from build123d import *

# Parameters (mm, degrees)
SKETCH1_R                = 57.5
SKETCH1_R_2              = 1.89865
SKETCH1_R_3              = 1.9939
SKETCH1_R_4              = 8
BOSS_EXTRUDE1_DEPTH      = 6.35
CUT_EXTRUDE1_DEPTH       = 82.564836173
SKETCH3_W                = 6.35
SKETCH3_H                = 80
CUT_EXTRUDE3_DEPTH       = 82.564836173
CUT_EXTRUDE4_DEPTH       = 82.564836173
CUT_EXTRUDE6_DEPTH       = 82.564836173
FILLET1_R                = 2
CIRPATTERN1_COUNT        = 8
FILLET1_OF_CIRPATTERN1_R = 2
CUT_EXTRUDE7_DEPTH       = 10
FILLET2_R                = 2
CIRPATTERN2_COUNT        = 8
FILLET2_OF_CIRPATTERN2_R = 2


with BuildPart() as part:
    # Sketch1 → Boss-Extrude1 (new body)
    with BuildSketch(Plane.XY):
        Circle(SKETCH1_R)
        with Locations((45.315389352, 21.130913087)):
            Circle(SKETCH1_R_2, mode=Mode.SUBTRACT)
        with Locations((46.467376211, -18.460307366)):
            Circle(SKETCH1_R_3, mode=Mode.SUBTRACT)
        Circle(SKETCH1_R_4, mode=Mode.SUBTRACT)
        with Locations((49.978847504, 1.454235937)):
            Circle(SKETCH1_R_3, mode=Mode.SUBTRACT)
        with Locations((0, -40)):
            Circle(SKETCH1_R_3, mode=Mode.SUBTRACT)
        with Locations((0, -50)):
            Circle(SKETCH1_R_2, mode=Mode.SUBTRACT)
        with Locations((-28.284271247, -28.284271247)):
            Circle(SKETCH1_R_3, mode=Mode.SUBTRACT)
        with Locations((-35.355339059, -35.355339059)):
            Circle(SKETCH1_R_2, mode=Mode.SUBTRACT)
        with Locations((-40, 0)):
            Circle(SKETCH1_R_3, mode=Mode.SUBTRACT)
        with Locations((-50, 0)):
            Circle(SKETCH1_R_2, mode=Mode.SUBTRACT)
        with Locations((-28.284271247, 28.284271247)):
            Circle(SKETCH1_R_3, mode=Mode.SUBTRACT)
        with Locations((-35.355339059, 35.355339059)):
            Circle(SKETCH1_R_2, mode=Mode.SUBTRACT)
        with Locations((0, 40)):
            Circle(SKETCH1_R_3, mode=Mode.SUBTRACT)
        with Locations((0, 50)):
            Circle(SKETCH1_R_2, mode=Mode.SUBTRACT)
        with Locations((35.355339059, -35.355339059)):
            Circle(SKETCH1_R_2, mode=Mode.SUBTRACT)
    extrude(amount=BOSS_EXTRUDE1_DEPTH)

    # Sketch2 → Cut-Extrude1 (cut, through all)
    with BuildSketch(Plane.XY):
        Polygon((12.5, -29.35), (41, -29.35), (41, 10.65), (44.5, 10.65), (44.5, 17), (41, 17), (41, 32), (21, 32), (21, 17), (17.5, 17), (17.5, 10.65), (21, 10.65), (21, 5.65), (12.5, 5.65), align=None)
    extrude(amount=CUT_EXTRUDE1_DEPTH, mode=Mode.SUBTRACT)

    # Sketch3 → Cut-Extrude3 (cut, through all)
    with BuildSketch(Plane.XY.offset(6.35)):
        with Locations((31, 32)):
            Rectangle(SKETCH3_W, SKETCH3_H)
    extrude(amount=-CUT_EXTRUDE3_DEPTH, mode=Mode.SUBTRACT)

    # Sketch4 → Cut-Extrude4 (cut, through all)
    with BuildSketch(Plane.XY.offset(6.35)):
        with BuildLine():
            Line((21, -36.5), (21, -16.443021443))
            Line((21, -16.443021443), (24.175, -16.470277755))
            Line((24.175, -16.470277755), (24.175, -57.5))
            Line((24.175, -57.5), (0, -57.5))
            ThreePointArc((0, -57.5), (14.849242405, -51.349242405), (21, -36.5))
        make_face()
        with BuildLine():
            Line((0, 57.5), (24.175, 57.5))
            Line((24.175, 57.5), (24.175, 16.470277755))
            Line((24.175, 16.470277755), (21, 16.443021443))
            Line((21, 16.443021443), (21, 36.5))
            ThreePointArc((21, 36.5), (14.849242405, 51.349242405), (0, 57.5))
        make_face()
    extrude(amount=-CUT_EXTRUDE4_DEPTH, mode=Mode.SUBTRACT)


with BuildPart() as cut_extrude4_kept_piece:
    # of the separate pieces the step leaves, the one the design keeps (cut_extrude4_pieces_kept)
    add(part.part.solids().sort_by_distance((0, 57.5, 0))[0])

    # Sketch6 → Cut-Extrude6 (cut, through all)
    with BuildSketch(Plane.XY.offset(6.35)):
        with BuildLine():
            Line((-13.691998588, 3.668759964), (-32.503404055, 8.709260868))
            ThreePointArc((-32.503404055, 8.709260868), (-33.65, 0), (-32.503404055, -8.709260868))
            Line((-32.503404055, -8.709260868), (-13.691998588, -3.668759964))
            ThreePointArc((-13.691998588, -3.668759964), (-14.175, 0), (-13.691998588, 3.668759964))
        make_face()
    cut_extrude6 = extrude(amount=-CUT_EXTRUDE6_DEPTH, mode=Mode.SUBTRACT)

    # Fillet1
    fillet1_edges = [cut_extrude4_kept_piece.edges().sort_by_distance(p)[0] for p in [
        (-13.691998588, 3.668759964, 3.175),
        (-13.691998588, -3.668759964, 3.175),
        (-32.503404055, -8.709260868, 3.175),
        (-32.503404055, 8.709260868, 3.175),
    ]]
    fillet(fillet1_edges, radius=FILLET1_R)

    # CirPattern1: Cut-Extrude6 ×8 about axis, 3 skipped
    cirpattern1_axis = Axis((0, 0, 0), (0, 0, -1))
    add([cut_extrude6.rotate(cirpattern1_axis, i * 360 / CIRPATTERN1_COUNT) for i in range(1, CIRPATTERN1_COUNT) if i not in (3, 4, 5)], mode=Mode.SUBTRACT)

    # Fillet1 of CirPattern1
    fillet1_of_cirpattern1_edges = [cut_extrude4_kept_piece.edges().sort_by_distance(p)[0] for p in [
        (-7.0875, 12.275910099, 3.175),
        (-12.275910099, 7.0875, 3.175),
        (-29.141754837, 16.825, 3.175),
        (-16.825, 29.141754837, 3.175),
        (3.668759964, 13.691998588, 3.175),
        (-3.668759964, 13.691998588, 3.175),
        (-8.709260868, 32.503404055, 3.175),
        (8.709260868, 32.503404055, 3.175),
        (-3.668759964, -13.691998588, 3.175),
        (3.668759964, -13.691998588, 3.175),
        (8.709260868, -32.503404055, 3.175),
        (-8.709260868, -32.503404055, 3.175),
        (-12.275910099, -7.0875, 3.175),
        (-7.0875, -12.275910099, 3.175),
        (-16.825, -29.141754837, 3.175),
        (-29.141754837, -16.825, 3.175),
    ]]
    fillet(fillet1_of_cirpattern1_edges, radius=FILLET1_OF_CIRPATTERN1_R)

    # Sketch7 → Cut-Extrude7 (cut)
    with BuildSketch(Plane.XY.offset(6.35)):
        with BuildLine():
            Line((-43.098920211, 33.070964631), (-29.215236756, 22.417639623))
            ThreePointArc((-29.215236756, 22.417639623), (-34.021863785, 14.092317397), (-36.50995702, 4.806627029))
            Line((-36.50995702, 4.806627029), (-53.860242094, 7.090835392))
            ThreePointArc((-53.860242094, 7.090835392), (-50.189755604, 20.789277463), (-43.098920211, 33.070964631))
        make_face()
    cut_extrude7 = extrude(amount=-CUT_EXTRUDE7_DEPTH, mode=Mode.SUBTRACT)

    # Fillet2
    fillet2_edges = [cut_extrude4_kept_piece.edges().sort_by_distance(p)[0] for p in [
        (-29.215236756, 22.417639623, 3.175),
        (-36.50995702, 4.806627029, 3.175),
        (-53.860242094, 7.090835392, 3.175),
        (-43.098920211, 33.070964631, 3.175),
    ]]
    fillet(fillet2_edges, radius=FILLET2_R)

    # CirPattern2: Cut-Extrude7 ×8 about axis, 4 skipped
    cirpattern2_axis = Axis((0, 0, 0), (0, 0, -1))
    add([cut_extrude7.rotate(cirpattern2_axis, i * 360 / CIRPATTERN2_COUNT) for i in range(1, CIRPATTERN2_COUNT) if i not in (2, 3, 4, 5)], mode=Mode.SUBTRACT)

    # Fillet2 of CirPattern2
    fillet2_of_cirpattern2_edges = [cut_extrude4_kept_piece.edges().sort_by_distance(p)[0] for p in [
        (-4.806627029, 36.50995702, 3.175),
        (-22.417639623, 29.215236756, 3.175),
        (-33.070964631, 43.098920211, 3.175),
        (-7.090835392, 53.860242094, 3.175),
        (-22.417639623, -29.215236756, 3.175),
        (-4.806627029, -36.50995702, 3.175),
        (-7.090835392, -53.860242094, 3.175),
        (-33.070964631, -43.098920211, 3.175),
        (-36.50995702, -4.806627029, 3.175),
        (-29.215236756, -22.417639623, 3.175),
        (-43.098920211, -33.070964631, 3.175),
        (-53.860242094, -7.090835392, 3.175),
    ]]
    fillet(fillet2_of_cirpattern2_edges, radius=FILLET2_OF_CIRPATTERN2_R)


solid = cut_extrude4_kept_piece.part
Input: part model. Units: mm. Frame: model coordinates. A direction names the side the tool comes from. Round coordinates to 2 decimals unless told otherwise and drop trailing zeros. Order: outer loops, then holes, each group sorted by start corner. A loop starts at its lowest first (then second) coordinate and runs counter-clockwise, first axis right, second up. Notation, with made-up numbers: (84.5, -25.5) - (92.5, -25.5) arc R21 cw to (92.5, -16.5) - close; hole circle Ø5 at (38, 48.5). An arc over 180 degrees is marked (long way). Use a Markdown table: item, result.
1. First-contact query: pin 1 (1.9 mm diameter, centred on y = 14.5, z = 2.5, fed in from +X); pin 2 (1.9 mm diameter, centred on x = 17.5, z = 2, fed in from -Y); pin 3 (1.5 mm diameter, centred on x = -9.5, z = 3, fed in from -Y). Flat tips, straight axial feed; report the tip coordinate or a pass-through.
Evaluation:
| item | result |
|---|---|
| pin 1 | x = 17.5 |
| pin 2 | y = -49.43 |
| pin 3 | y = -56.83 |
2. Section A-A on y = -40. Return the cut outline in (x, z).
Evaluation:
| item | result |
|---|---|
| outline | (-41.31, 0) - (-30.69, 0) - (-30.69, 6.35) - (-41.31, 6.35) - close; (-5.27, 0) - (-1.99, 0) - (-1.99, 6.35) - (-5.27, 6.35) - close; (1.99, 0) - (20.71, 0) - (20.71, 6.35) - (1.99, 6.35) - close |
3. Access query for faces 1 (the face through (17.5, 14, 3)), 2 (the face through (-5.955, 45.234, 3.219)). Directions: +Z, -Z, +X, -X, +Y, -Y. A direction counts if a zero-diameter tool reaches every point of the face in a straight line with its end or side. Return the directions, or none.
Evaluation:
| item | result |
|---|---|
| face 1 | +Z, -Z, +X |
| face 2 | +Z, -Z |
4. Material intervals for probe 1 along X at (y, z) = (41.5, 5.5); probe 2 along X at (y, z) = (-4, 4); probe 3 along Y at (x, z) = (-12, 3.5), sorted ascending.
Evaluation:
| item | result |
|---|---|
| probe 1 | -39.8 to -31.84, -5.46 to -1.31, 1.31 to 20.4 |
| probe 2 | -57.36 to -33.41, -15.1 to -6.93, 6.93 to 12.5 |
| probe 3 | -56.23 to -52.98, -34.81 to -20.78, -7.97 to 7.97, 20.78 to 34.81, 52.98 to 56.23 |
5. Section D-D on z = 1. State how many separate pieces and enclosed holes the cut face has, then the cut area to 3 significant figures.
Evaluation:
| item | result |
|---|---|
| separate pieces | 1 |
| enclosed holes | 20 |
| area | 3,920 mm^2 |
6. Mould query, pull axis Y, two halves, no side actions, for faces 3 (the face through (-53.2, 7.64, 3.13)), 4 (the face through (-10, 1, 6.35)), 5 (the face through (-51.897, 0.083, 3.131)). Classes: +Y half, -Y half, draft (parallel to the pull), parting line (faces both ways), or undercut.
Evaluation:
| item | result |
|---|---|
| face 3 | undercut |
| face 4 | draft |
| face 5 | undercut |
7. Section B-B on x = -50. Return the cut outline in (y, z).
Evaluation:
| item | result |
|---|---|
| outline | (-28.39, 0) - (-21.24, 0) - (-21.24, 6.35) - (-28.39, 6.35) - close; (-6.58, 0) - (-1.9, 0) - (-1.9, 6.35) - (-6.58, 6.35) - close; (1.9, 0) - (6.58, 0) - (6.58, 6.35) - (1.9, 6.35) - close; (21.24, 0) - (28.39, 0) - (28.39, 6.35) - (21.24, 6.35) - close |
8. Section C-C on x = -40. Return the cut outline in (y, z), then the cut area to 3 significant figures.
Evaluation:
| item | result |
|---|---|
| outline | (-41.31, 0) - (-30.69, 0) - (-30.69, 6.35) - (-41.31, 6.35) - close; (-5.27, 0) - (-1.99, 0) - (-1.99, 6.35) - (-5.27, 6.35) - close; (1.99, 0) - (5.27, 0) - (5.27, 6.35) - (1.99, 6.35) - close; (30.69, 0) - (41.31, 0) - (41.31, 6.35) - (30.69, 6.35) - close |
| area | 176 mm^2 |
